Autodesk Inventor part; units mm, degrees
ref_plane "YZ Plane" through (0, 0, 0) normal (1, 0, 0) x (0, 1, 0)
ref_plane "XZ Plane" through (0, 0, 0) normal (0, 1, 0) x (-1, 0, 0)
ref_plane "XY Plane" through (0, 0, 0) normal (0, 0, 1) x (1, 0, 0)
sketch "Boceto1" plane through (0, 0, 0) normal (0, 1, 0) x (-1, 0, 0)
  line L0 (27.5, 50) -> (-27.5, 50)
  line L1 (-27.5, 50) -> (-27.5, -50)
  line L2 (-27.5, -50) -> (27.5, -50)
  line L3 (27.5, -50) -> (27.5, 50)
  line L4 (27.5, 50) -> (-27.5, -50) construction
  line L5 (-27.5, 50) -> (27.5, -50) construction
  point P0 (0, 0)
  dimension "d0" = 55
  dimension "d1" = 100
extrude "Extrusión1" add sketch "Boceto1" along normal blind 30
sketch "Boceto2" plane through (27.5, 0, -50) normal (0, 0, -1) x (-1, 0, 0)
  line L0 (10, 25) -> (20, 25)
  line L1 (20, 25) -> (20, 15)
  line L2 (20, 15) -> (10, 15)
  line L3 (10, 15) -> (10, 25)
  line L4 (10, 25) -> (20, 15) construction
  line L5 (20, 25) -> (10, 15) construction
  line L6 (0, 30) -> (55, 30)
  line L7 (0, 0) -> (0, 30)
  point P0 (27.5, 0)
  point P1 (15, 20)
  point P2 (15, 25)
  dimension "d4" = 10
  dimension "d5" = 10
  dimension "d6" = 5
  dimension "d7" = 10
extrude "Extrusión2" add sketch "Boceto2" along normal blind 10
sketch "Boceto3" plane through (-27.5, 0, 50) normal (0, 0, 1) x (1, 0, 0)
  circle A0 centre (27.5, 20) radius 5
  line L0 (0, 30) -> (55, 30)
  point P0 (27.5, 0)
  point P1 (27.5, 30)
  dimension "d10" = 10
  dimension "d11" = 10
extrude "Extrusión3" cut sketch "Boceto3" against normal blind 15
sketch "Boceto4" plane through (0, 30, 0) normal (0, 1, 0) x (1, 0, 0)
  line L0 (-20, 23) -> (20, 23)
  line L1 (20, 23) -> (20, -23)
  line L2 (20, -23) -> (-20, -23)
  line L3 (-20, -23) -> (-20, 23)
  line L4 (-20, 23) -> (20, -23) construction
  line L5 (20, 23) -> (-20, -23) construction
  point P0 (0, 0)
  dimension "d14" = 40
  dimension "d15" = 46
extrude "Extrusión4" cut sketch "Boceto4" against normal blind 20
properties part number "camera_support_2"
Verification items for the finished model (mm, model axes). A direction names the side the tool comes from. Coordinates: 2 decimals unless noted, no trailing zeros. Order: outer loops, then holes, each group sorted by start corner. A loop starts at its lowest first (then second) coordinate and runs counter-clockwise, first axis right, second up. Notation, with made-up numbers: (-20, 43.25) -> (19, 43.25) arc R8 cw to (19, 58.25) -> close; hole circle Ø8 at (-15, 65). An arc over 180 degrees is marked (long way). Answer as CSV lines item,"result". Start each with the question number.
1) Release check for a two-part mould opening along X. For faces 6 (the face through (7.5, 20, -55)), 7 (the face through (25, 30, 1)), 8 (the face through (0, 10, 0)) record: released by +X, released by -X, zero draft, split by the parting line, or undercut.
2) Cross-section at D-D, the plane y = 20. Record the boundary of the cut face in (x, z).
3) Cross-section at B-B, the plane x = 0. Record the boundary of the cut face in (y, z), then the cut area to 3 significant figures.
4) Cross-section at A-A, the plane y = 27. Record the boundary of the cut face in (x, z), then the cut area to 3 significant figures.
5) Cross-section at C-C, the plane z = -9.5. Record the boundary of the cut face in (x, y).
6) Material ranges on L1, parallel to Z at x = -14.5, y = 12.5; L2, parallel to Y at x = 0, z = 40.5; L3, parallel to X at y = 12.75, z = -12, recorded low to high. Write a range as [from, to].
7) Gauge pin test, flat ends, axial feed: pin 1 Ø5 at (x, z) = (11.5, -53.5) entering from -Y; pin 2 Ø9 at (x, y) = (0, 20) entering from +Z; pin 3 Ø6 at (x, z) = (-7.5, -5) entering from +Y. Record the tip position at first contact, or that the pin passes through.
8) Set-up check for faces 1 (the face through (0, 20, 35)), 2 (the face through (13, 25, -55)), 3 (the face through (0, 20, 23)), 4 (the face through (17.5, 20, -55)), 5 (the face through (12, 15, -55)): record each of +Z, -Z, +X, -X, +Y, -Y from which the full face is reachable in a straight line by a thin tool's end or side.
Conclusion:
1,face 6,"released by -X"
1,face 7,"zero draft"
1,face 8,"undercut"
2,outline,"(-27.5, -50) -> (7.5, -50) -> (7.5, -60) -> (17.5, -60) -> (17.5, -50) -> (27.5, -50) -> (27.5, 50) -> (5, 50) -> (5, 35) -> (-5, 35) -> (-5, 50) -> (-27.5, 50) -> close; hole (-20, -23) -> (20, -23) -> (20, 23) -> (-20, 23) -> close"
3,outline,"(0, -50) -> (30, -50) -> (30, -23) -> (10, -23) -> (10, 23) -> (30, 23) -> (30, 50) -> (25, 50) -> (25, 35) -> (15, 35) -> (15, 50) -> (0, 50) -> close"
3,area,"1,930 mm²"
4,outline,"(-27.5, -50) -> (27.5, -50) -> (27.5, 50) -> (-27.5, 50) -> close; hole (-20, -23) -> (20, -23) -> (20, 23) -> (-20, 23) -> close"
4,area,"3,660 mm²"
5,outline,"(-27.5, 0) -> (27.5, 0) -> (27.5, 30) -> (20, 30) -> (20, 10) -> (-20, 10) -> (-20, 30) -> (-27.5, 30) -> close"
6,L1,"z = [-50, -23], [23, 50]"
6,L2,"y = [0, 15], [25, 30]"
6,L3,"x = [-27.5, -20], [20, 27.5]"
7,pin 1,"stops at y = 15"
7,pin 2,"stops at z = 35"
7,pin 3,"stops at y = 10"
8,face 1,"+Z"
8,face 2,"-Z, +X, -X, +Y"
8,face 3,"+Y"
8,face 4,"-Z, +X, +Y, -Y"
8,face 5,"-Z, +X, -X, -Y"
